Source: CAD feature listing. Evaluate the final solid. Frame: model axes, mm. A direction names the side the tool comes from. Give positions to 0.01 mm unless a question says otherwise; leave off trailing zeros. Loops run counter-clockwise (first coordinate to the right, second up) from the corner with the lowest first, then second, coordinate; pieces in that order, holes last. Notation, with made-up numbers: M 16.25,-37 L 31.25,-37 A7 ccw 31.25,-32 Z; hole C 44.5,-2 d3. An arc over 180 degrees is marked long. Answer in a Markdown table with one row per item.
```python
from build123d import *

# Parameters (mm, degrees)
BOSS_EXTRUDE1_DEPTH = 6.5


with BuildPart() as part:
    # Sketch1 → Boss-Extrude1 (new body)
    with BuildSketch(Plane(origin=(120.8182, 0, 0), x_dir=(0, 0, -1), z_dir=(1, 0, 0))):
        with BuildLine():
            Line((846.478661638, 494.561851817), (1040.702839036, 273.07651954))
            ThreePointArc((1040.702839036, 273.07651954), (1004.366479469, 90.186693697), (837.070444967, 172.533862824))
            Line((837.070444967, 172.533862824), (779.311502219, 461.398343217))
            ThreePointArc((779.311502219, 461.398343217), (800.164646921, 503.763471885), (846.478661638, 494.561851817))
        make_face()
        with BuildLine():
            Line((840.809621425, 489.590576019), (1035.033798823, 268.105243742))
            ThreePointArc((1035.033798823, 268.105243742), (1001.028357677, 96.947503035), (844.464091935, 174.012235074))
            Line((844.464091935, 174.012235074), (786.705149187, 462.876715467))
            ThreePointArc((786.705149187, 462.876715467), (803.502768714, 497.002662547), (840.809621425, 489.590576019))
        make_face(mode=Mode.SUBTRACT)
    extrude(amount=-BOSS_EXTRUDE1_DEPTH)


solid = part.part
```
Q1. Mould query, pull axis Z, two halves, no side actions, for faces 3 (the flat face through (117.614, 314.944, -808.595)), 4 (the cylindrical face through (117.61, 98.23, -1003.54)), 5 (the flat face through (114.318, 358, -957)). Classes: +Z half, -Z half, draft (parallel to the pull), parting line (faces both ways), or undercut.
Values follow:
| item | result |
|---|---|
| face 3 | +Z half |
| face 4 | undercut |
| face 5 | draft |
Q2. Section query B-B (z = -1022.5). Output: boundary loops of the cut face in (x, y), plus the area to 3 significant figures.
Values follow:
| item | result |
|---|---|
| outline | M 114.32,101.28 L 120.82,101.28 L 120.82,110.87 L 114.32,110.87 Z; M 114.32,282.4 L 120.82,282.4 L 120.82,293.83 L 114.32,293.83 Z |
| area | 137 mm^2 |
Q3. Section query C-C (x = 118.5). Output: boundary loops of the cut face in (y, z), plus the area to 3 significant figures.
Values follow:
| item | result |
|---|---|
| outline | M 172.53,-837.07 A117.54 ccw long 273.08,-1040.7 L 494.56,-846.48 A38.77 ccw 461.4,-779.31 Z; hole M 174.01,-844.46 A110 ccw long 268.11,-1035.03 L 489.59,-840.81 A31.23 ccw 462.88,-786.71 Z |
| area | 8,280 mm^2 |
Q4. Reachability of faces 1 (the flat face through (117.61, 380.4, -936.56)), 2 (the flat face through (120.818, 358, -957)) from +Z, -Z, +X, -X, +Y, -Y: full face, straight path, thin tool, end or side. Return the list, or none.
Values follow:
| item | result |
|---|---|
| face 1 | +X, -X |
| face 2 | +Z, -Z, +X, +Y, -Y |
Q5. Contact query for flat-ended pins moving along their axis: pin 1 Ø1 at (x, z) = (117, -842.5) entering from +Y; pin 2 Ø1 at (x, z) = (118, -1002.5) entering from -Y; pin 3 Ø1 at (x, y) = (120, 462) entering from -Z. Output: stop coordinate, or through.
Values follow:
| item | result |
|---|---|
| pin 1 | y = 498.91 |
| pin 2 | y = 89.05 |
| pin 3 | z = -875.47 |
Q6. Section query A-A (y = 248.5). Output: boundary loops of the cut face in (x, z), plus the area to 3 significant figures.
Values follow:
| item | result |
|---|---|
| outline | M 114.32,-1057.28 L 120.82,-1057.28 L 120.82,-1048.76 L 114.32,-1048.76 Z; M 114.32,-829.57 L 120.82,-829.57 L 120.82,-821.88 L 114.32,-821.88 Z |
| area | 105 mm^2 |
Q7. Ray query, probe 1 along Z at (x, y) = (116.75, 195.58); probe 2 along Z at (x, y) = (118.5, 118); probe 3 along Y at (x, z) = (118.75, -1026). Return the intervals inside material, ascending. Write a range as from..to.
Values follow:
| item | result |
|---|---|
| probe 1 | -1069.87..-1062.33, -840.15..-832.46 |
| probe 2 | -1040.63..-1030.31, -874.35..-864.03 |
| probe 3 | 103.99..113.89, 278.41..289.84 |
